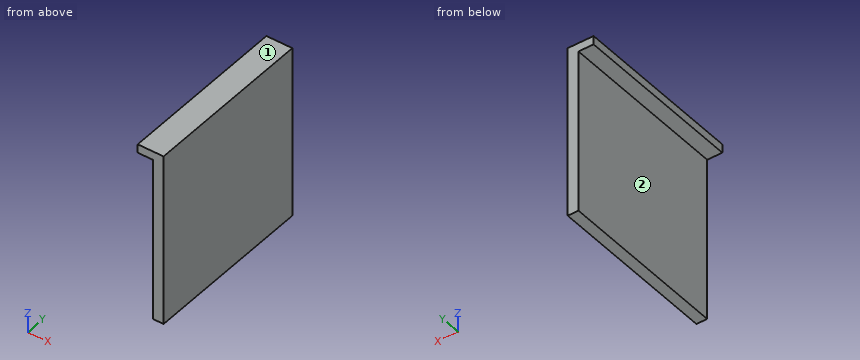
Solid Edge part; units mm, degrees
sketch "Sketch1" plane through (0, 0, 0) normal (0, -1, 0) x (1, 0, 0)
  line L0 (0, 0) -> (0, 20)
  line L1 (0, 20) -> (-3, 20)
  line L2 (-3, 20) -> (-3, 19)
  line L3 (-3, 19) -> (-1.25, 19)
  line L4 (-1.25, 19) -> (-1.25, 0)
  line L5 (-1.25, 0) -> (0, 0)
extrude "Protrusion1" add sketch "Sketch1" against normal blind 20
Source: CAD feature listing. Evaluate the final solid. Frame: model axes, mm. Face numbers are marked on the shaded views. A direction names the side the tool comes from. Coordinates: 2 decimals unless noted, no trailing zeros. Loops run counter-clockwise (first coordinate to the right, second up) from the corner with the lowest first, then second, coordinate; pieces in that order, holes last. Notation, with made-up numbers: M -27.75,74.25 L -9.75,74.25 A21 cw -9.75,80.25 Z; hole C -12,68.5 d2. An arc over 180 degrees is marked long. Put each result on its own line as item: value. Start each with the question number.
1) Cut plane A-A on y = 14.25. Return the cut outline in (x, z), then the cut area to 4 significant figures.
2) Contact query for flat-ended pins moving along their axis: pin 1 Ø1.4 at (x, y) = (-2, 5) entering from -Z; pin 2 Ø5 at (y, z) = (5.5, 3.5) entering from -X. Output: stop coordinate, or through.
3) Cut plane C-C on z = 15.75. Return the cut outline in (x, y).
4) Ray query, L1, parallel to X at y = 15.5, z = 3.25; L2, parallel to Z at x = -2.25, y = 4.75. Return the intervals inside material, ascending. Write a range as from..to.
5) Cut plane B-B on x = -2.6. Return the cut outline in (y, z), then the cut area to 3 significant figures.
6) Reachability of the marked faces 1 and 2 from +Z, -Z, +X, -X, +Y, -Y: full face, straight path, thin tool, end or side. Return the list, or none.
The answers:
1. outline: M -3,19 L -1.25,19 L -1.25,0 L 0,0 L 0,20 L -3,20 Z
1. area: 26.75 mm²
2. pin 1: stops at z = 19
2. pin 2: stops at x = -1.25
3. outline: M -1.25,0 L 0,0 L 0,20 L -1.25,20 Z
4. L1: x = -1.25..0
4. L2: z = 19..20
5. outline: M 0,19 L 20,19 L 20,20 L 0,20 Z
5. area: 20.0 mm²
6. face 1: +Z, +X, -X, +Y, -Y
6. face 2: -Z, -X, +Y, -Y
